```python
from build123d import *

# Parameters (mm, degrees)
F0_R      = 3.5
F0_R_2    = 7
F1_DEPTH  = 25
F3_DEPTH  = 10
F5_D      = 13
F6_W      = 36
F6_H      = 15
F6_H_2    = 20
F7_DEPTH  = 30.001
F8_W      = 30
F8_H      = 5
F9_DEPTH  = 80.001
F10_W     = 50
F10_H     = 10
F11_DEPTH = 10
F13_DEPTH = 10


with BuildPart() as f1:
    # F0 (on Right) → F1 (new body, symmetric)
    with BuildSketch(Plane.YZ):
        with BuildLine():
            Line((0, 15), (0, 0))
            Line((0, 0), (55, 0))
            Line((55, 0), (55, 10))
            Line((55, 10), (30, 10))
            Line((30, 10), (30, 45))
            ThreePointArc((30, 45), (8.291796, 58.416408), (6, 33))
            Line((6, 33), (6, 15))
            Line((6, 15), (0, 15))
        make_face()
        with Locations((18, 10)):
            Circle(F0_R, mode=Mode.SUBTRACT)
        with Locations((15, 45)):
            Circle(F0_R_2, mode=Mode.SUBTRACT)
    extrude(amount=F1_DEPTH, both=True)

    # F2 (on face) → F3 (join)
    with BuildSketch(Plane(origin=(0, 0, 0), x_dir=(1, 0, 0), z_dir=(0, 0, -1))):
        with BuildLine():
            Line((25, -55), (-25, -55))
            ThreePointArc((-25, -55), (0, -80), (25, -55))
        make_face()
    extrude(amount=-F3_DEPTH)

    # F5 (through all)
    with Locations(Plane.XY.offset(10)):
        with Locations((0, 55)):
            Hole(F5_D / 2)

    # F6 (on face) → F7 (cut, through all)
    with BuildSketch(Plane(origin=(0, 30, 0), x_dir=(-1, 0, 0), z_dir=(0, 1, 0))):
        with Locations((0, 52.5)):
            Rectangle(F6_W, F6_H)
        with Locations((0, 35)):
            Rectangle(F6_W, F6_H_2)
    extrude(amount=-F7_DEPTH, mode=Mode.SUBTRACT)

    # F8 (on face) → F9 (cut, through all)
    with BuildSketch(Plane.XZ):
        with Locations((0, 2.5)):
            Rectangle(F8_W, F8_H)
        with Locations((0, -2.5)):
            Rectangle(F8_W, F8_H)
    extrude(amount=-F9_DEPTH, mode=Mode.SUBTRACT)

    # F10 (on face) → F11 (join)
    with BuildSketch(Plane(origin=(0, 30, 0), x_dir=(-1, 0, 0), z_dir=(0, 1, 0))):
        with Locations((0, 15)):
            Rectangle(F10_W, F10_H)
    extrude(amount=F11_DEPTH)

    # F12 (on face) → F13 (cut)
    with BuildSketch(Plane(origin=(0, 40, 0), x_dir=(-1, 0, 0), z_dir=(0, 1, 0))):
        with BuildLine():
            ThreePointArc((0, 10), (7.071068, 12.928932), (10, 20))
            Line((10, 20), (-10, 20))
            ThreePointArc((-10, 20), (-7.071068, 12.928932), (0, 10))
        make_face()
    extrude(amount=-F13_DEPTH, mode=Mode.SUBTRACT)


solid = f1.part
```
The model under review builds one solid part; all positions refer to its coordinate system, in mm. A direction names the side the tool comes from. Coordinates: 2 decimals unless noted, no trailing zeros. Order: outer loops, then holes, each group sorted by start corner. A loop starts at its lowest first (then second) coordinate and runs counter-clockwise, first axis right, second up. Notation, with made-up numbers: (-37.75, 8) -> (-14.75, 8) arc R31 ccw to (-14.75, 34) -> close; hole circle Ø7 at (-12.75, 13). An arc over 180 degrees is marked (long way). Answer in a Markdown table with one row per item. Add a question column.
Item 1: We need section D-D on y = 18. Write out the cut boundary in (x, z).
Item 2: We need section C-C on z = 11. Write out the cut boundary in (x, y).
Item 3: We need section B-B on z = 40.5. Write out the cut boundary in (x, y), plus the area to 3 significant figures.
Item 4: Machinability: for faces 1 (the flat face through (-18, 19, 38)), 2 (the flat face through (5, 60, 10)), 3 (the flat face through (-1.7, 30, 24.8)), 4 (the cylindrical face through (21.45, 14.09, 51.94)), 5 (the flat face through (0, 3, 15)), which of the approach directions +Z, -Z, +X, -X, +Y, -Y give a long, thin tool a straight path to every point of the face, cutting with its end or side? Answer none if there is none.
Item 5: Mouldability with a two-part tool opening along X and no side actions: class faces 6 (the flat face through (0, 6, 22)), 7 (the flat face through (15, 37, 2)), 8 (the flat face through (-25, 21, 23)) as +X half, -X half, draft (parallel to the pull), parting line (faces both ways), or undercut.
Item 6: We need section A-A on y = 32.5. Write out the cut boundary in (x, z), plus the area to 3 significant figures.
Item 7: Clearance check with flat-ended pins moving along their axes: pin 1 (6 mm diameter, centred on x = -14, z = 31.5, fed in from +Y); pin 2 (3 mm diameter, centred on x = -18.5, y = 8, fed in from +Z); pin 3 (17 mm diameter, centred on x = 0, y = 55, fed in from +Z); pin 4 (2 mm diameter, centred on x = -3, y = 13.5, fed in from -Z). State where each tip first meets the part, or that it passes through.
Item 8: To check wall thickness, follow probe 1 along Y at (x, z) = (20.25, 45); probe 2 along X at (y, z) = (26.5, 31.5); probe 3 along X at (y, z) = (7, 3). State the ranges of each line that lie inside material, in increasing order.
Final values:
| question | item | result |
|---|---|---|
| 1 | outline | (-25, 0) -> (-15, 0) -> (-15, 5) -> (15, 5) -> (15, 0) -> (25, 0) -> (25, 6.5) -> (-25, 6.5) -> close; (-25, 13.5) -> (25, 13.5) -> (25, 38.68) -> (18, 38.68) -> (18, 25) -> (-18, 25) -> (-18, 38.68) -> (-25, 38.68) -> close; (-25, 51.32) -> (-18, 51.32) -> (-18, 59.7) -> (-25, 59.7) -> close; (18, 51.32) -> (25, 51.32) -> (25, 59.7) -> (18, 59.7) -> close |
| 2 | outline | (-25, 0) -> (25, 0) -> (25, 14.65) -> (-25, 14.65) -> close; (-25, 21.35) -> (25, 21.35) -> (25, 40) -> (4.36, 40) -> (4.36, 30) -> (-4.36, 30) -> (-4.36, 40) -> (-25, 40) -> close |
| 3 | outline | (-25, 0.69) -> (-18, 0.69) -> (-18, 9.64) -> (-25, 9.64) -> close; (-25, 20.36) -> (-18, 20.36) -> (-18, 30) -> (-25, 30) -> close; (18, 0.69) -> (25, 0.69) -> (25, 9.64) -> (18, 9.64) -> close; (18, 20.36) -> (25, 20.36) -> (25, 30) -> (18, 30) -> close |
| 3 | area | 260 mm2 |
| 4 | face 1 | +Z, +Y, -Y |
| 4 | face 2 | +Z, +X, -X, +Y |
| 4 | face 3 | +Z, +Y |
| 4 | face 4 | +X, -X |
| 4 | face 5 | +X, -X, -Y |
| 5 | face 6 | draft |
| 5 | face 7 | undercut |
| 5 | face 8 | -X half |
| 6 | outline | (-25, 0) -> (-15, 0) -> (-15, 5) -> (15, 5) -> (15, 0) -> (25, 0) -> (25, 20) -> (10, 20) arc R10 cw to (0, 10) arc R10 cw to (-10, 20) -> (-25, 20) -> close |
| 6 | area | 693 mm2 |
| 7 | pin 1 | passes through |
| 7 | pin 2 | stops at z = 58.96 |
| 7 | pin 3 | stops at z = 10 |
| 7 | pin 4 | stops at z = 5 |
| 8 | probe 1 | y = 0 to 8, 22 to 30 |
| 8 | probe 2 | x = -25 to -18, 18 to 25 |
| 8 | probe 3 | x = -25 to -15, 15 to 25 |
